Autodesk Inventor part; units mm, degrees
ref_plane "YZ Plane" through (0, 0, 0) normal (1, 0, 0) x (0, 1, 0)
ref_plane "XZ Plane" through (0, 0, 0) normal (0, 1, 0) x (-1, 0, 0)
ref_plane "XY Plane" through (0, 0, 0) normal (0, 0, 1) x (1, 0, 0)
sketch "Sketch1" plane through (0, 0, 0) normal (0, 0, 1) x (1, 0, 0)
  line L0 (-53.3927, 155.3954) -> (-51.1476, 153.1504) construction
  line L1 (-53.3927, 155.3954) -> (-73.3092, 135.4789) construction
  line L2 (-73.3092, 135.4789) -> (-71.0641, 133.2339) construction
  line L3 (-71.0641, 133.2339) -> (-51.1476, 153.1504) construction
  line L4 (-46.6575, 157.6405) -> (-51.1476, 153.1504) construction
  line L5 (-46.6575, 157.6405) -> (-48.9026, 159.8856) construction
  line L6 (-53.3927, 155.3954) -> (-48.9026, 159.8856) construction
  line L7 (-59.8388, 148.9493) -> (-66.574, 155.6845)
  line L8 (-66.574, 155.6845) -> (-48.6135, 173.645)
  line L9 (-48.6135, 173.645) -> (-30.653, 155.6845)
  line L10 (-30.653, 155.6845) -> (-62.0839, 124.2536)
  line L11 (-62.0839, 124.2536) -> (-71.0641, 133.2339)
  line L12 (-59.8388, 148.9493) -> (-48.9026, 159.8856)
  line L13 (-48.9026, 159.8856) -> (-46.6575, 157.6405)
  line L14 (-46.6575, 157.6405) -> (-71.0641, 133.2339)
  circle A0 centre (-59.164, 136.1538) radius 3.3782
  point P0 (0, 0)
  dimension "d7" = 44.45
  dimension "d8" = 25.4
  dimension "d9" = 25.4
  dimension "d10" = 12.7
extrude "Extrusion1" add sketch "Sketch1" along normal blind 3.175
fillet "Fillet1" radius 3.175 6 edges at (-62.0839, 124.2536, 1.5875) (-59.8388, 148.9493, 1.5875) (-66.574, 155.6845, 1.5875) (-71.0641, 133.2339, 1.5875) (-48.6135, 173.645, 1.5875) (-30.653, 155.6845, 1.5875)
properties part number "V5 Conveyor Plate Bracket P3" material "Aluminum-6061"
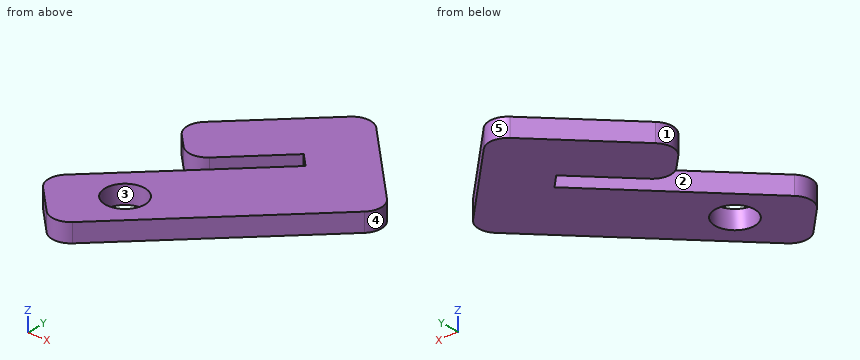
The listing builds one solid part. Answer for the finished solid, in the listing's coordinates (mm). Face numbers are marked on the shaded views. A direction names the side the tool comes from. Coordinates: 2 decimals unless noted, no trailing zeros. Loops run counter-clockwise (first coordinate to the right, second up) from the corner with the lowest first, then second, coordinate; pieces in that order, holes last. Notation, with made-up numbers: (84.25, -27.5) - (123.25, -27.5) arc R23 ccw to (123.25, -10.5) - close; hole circle Ø2 at (3.25, 84). An arc over 180 degrees is marked (long way). Use a Markdown table: item, result. Add a question column.
1) Find the intervals of material crossed by line 1 (Y direction, x = -59, z = 2.4); line 2 (Y direction, x = -60, z = 0.7); line 3 (Y direction, x = -54, z = 2.7), in increasing order.
2) The mould has two halves that part along X. Classify the marked faces 3, 4 and 5: released by +X, released by -X, zero draft, split by the parting line, or undercut.
3) Given pin 1 (10 mm diameter, centred on x = -38, y = 167.5, fed in from +Z) (3 decimals); pin 2 (1 mm diameter, centred on x = -60, z = 1, fed in from +Y), each flat-ended and moving along its own axis, determine where each tip first touches the part or whether it passes through.
4) The part is cut by section D-D, the plane x = -39. Give the vertices of the cut face in (y, z) (1 decimal).
5) The part is cut by section B-B, the plane y = 152.5. Give the vertices of the cut face in (x, z) (1 decimal).
6) For the marked faces 1 and 2, determine the directions among +Z, -Z, +X, -X, +Y, -Y from which every point of the face is accessible in a straight line to the end or side of a thin tool.
7) The part is cut by section A-A, the plane x = -51.5. Give the vertices of the cut face in (y, z) (1 decimal).
Here are the results:
| question | item | result |
|---|---|---|
| 1 | line 1 | y = 127.34 to 132.78, 139.53 to 145.3, 150.38 to 163.26 |
| 1 | line 2 | y = 126.35 to 132.88, 139.43 to 144.3, 150.27 to 162.26 |
| 1 | line 3 | y = 132.34 to 150.3, 154.79 to 168.26 |
| 2 | face 3 | undercut |
| 2 | face 4 | released by +X |
| 2 | face 5 | split by the parting line |
| 3 | pin 1 | stops at z = 3.175 |
| 3 | pin 2 | stops at y = 162.76 |
| 4 | outline | (147.3, 0) - (164, 0) - (164, 3.2) - (147.3, 3.2) - close |
| 5 | outline | (-63.4, 0) - (-56.3, 0) - (-56.3, 3.2) - (-63.4, 3.2) - close; (-51.8, 0) - (-33.8, 0) - (-33.8, 3.2) - (-51.8, 3.2) - close |
| 6 | face 1 | +Z, -Z, -X |
| 6 | face 2 | +Z, -Z |
| 7 | outline | (134.8, 0) - (152.8, 0) - (152.8, 3.2) - (134.8, 3.2) - close; (157.3, 0) - (170.8, 0) - (170.8, 3.2) - (157.3, 3.2) - close |
